Part model, mm, in its own coordinate system. A direction names the side the tool comes from. Round coordinates to 2 decimals unless told otherwise and drop trailing zeros. Loops run counter-clockwise (first coordinate to the right, second up) from the corner with the lowest first, then second, coordinate; pieces in that order, holes last.
from build123d import *

# Parameters (mm, degrees)
BOSS_EXTRUDE1_DEPTH = 6.35


with BuildPart() as part:
    # Sketch1 → Boss-Extrude1 (new body)
    with BuildSketch(Plane(origin=(0, 0, 0), x_dir=(1, 0, 0), z_dir=(0, 1, 0))):
        with BuildLine():
            Line((-79.362966154, -13.293541536), (-79.362966154, -21.341955347))
            Line((-79.362966154, -21.341955347), (-76.187966154, -21.341955347))
            Line((-76.187966154, -21.341955347), (-76.187966154, -19.589355347))
            Line((-76.187966154, -19.589355347), (-73.647966154, -19.589355347))
            Line((-73.647966154, -19.589355347), (-73.647966154, -21.341955347))
            Line((-73.647966154, -21.341955347), (-72.377966154, -21.341955347))
            Line((-72.377966154, -21.341955347), (-72.377966154, -24.389814703))
            Line((-72.377966154, -24.389814703), (-73.647966154, -24.389814703))
            Line((-73.647966154, -24.389814703), (-73.647966154, -26.142414703))
            Line((-73.647966154, -26.142414703), (-76.187966154, -26.142414703))
            Line((-76.187966154, -26.142414703), (-76.187966154, -24.389814703))
            Line((-76.187966154, -24.389814703), (-79.362966154, -24.389814703))
            Line((-79.362966154, -24.389814703), (-79.362966154, -32.343541536))
            Line((-79.362966154, -32.343541536), (-85.712966154, -32.343541536))
            Line((-85.712966154, -32.343541536), (-85.712966154, -38.693541536))
            Line((-85.712966154, -38.693541536), (-79.362966154, -38.693541536))
            Line((-79.362966154, -38.693541536), (-47.528264268, -38.693541536))
            Line((-47.528264268, -38.693541536), (-47.528264268, -35.518541536))
            Line((-47.528264268, -35.518541536), (-49.280864268, -35.518541536))
            Line((-49.280864268, -35.518541536), (-49.280864268, -32.978541536))
            Line((-49.280864268, -32.978541536), (-47.528264268, -32.978541536))
            Line((-47.528264268, -32.978541536), (-47.528264268, -31.708541536))
            Line((-47.528264268, -31.708541536), (-44.480404912, -31.708541536))
            Line((-44.480404912, -31.708541536), (-44.480404912, -32.978541536))
            Line((-44.480404912, -32.978541536), (-42.727804912, -32.978541536))
            Line((-42.727804912, -32.978541536), (-42.727804912, -35.518541536))
            Line((-42.727804912, -35.518541536), (-44.480404912, -35.518541536))
            Line((-44.480404912, -35.518541536), (-44.480404912, -38.693541536))
            Line((-44.480404912, -38.693541536), (20.734235732, -38.693541536))
            Line((20.734235732, -38.693541536), (20.734235732, -35.518541536))
            Line((20.734235732, -35.518541536), (18.981635732, -35.518541536))
            Line((18.981635732, -35.518541536), (18.981635732, -32.978541536))
            Line((18.981635732, -32.978541536), (20.734235732, -32.978541536))
            Line((20.734235732, -32.978541536), (20.734235732, -31.708541536))
            Line((20.734235732, -31.708541536), (23.782095088, -31.708541536))
            Line((23.782095088, -31.708541536), (23.782095088, -32.978541536))
            Line((23.782095088, -32.978541536), (25.534695088, -32.978541536))
            Line((25.534695088, -32.978541536), (25.534695088, -35.518541536))
            Line((25.534695088, -35.518541536), (23.782095088, -35.518541536))
            Line((23.782095088, -35.518541536), (23.782095088, -38.693541536))
            Line((23.782095088, -38.693541536), (79.387033846, -38.693541536))
            ThreePointArc((79.387033846, -38.693541536), (1.583968625, -14.958867645), (-79.362966154, -6.943541536))
            Line((-79.362966154, -6.943541536), (-85.712966154, -6.943541536))
            Line((-85.712966154, -6.943541536), (-85.712966154, -13.293541536))
            Line((-85.712966154, -13.293541536), (-79.362966154, -13.293541536))
        make_face()
    extrude(amount=BOSS_EXTRUDE1_DEPTH)


solid = part.part
1) Slice it at B-B, the plane z = 10. Give the cut face in (x, y), then the cut area to 3 significant figures.
Values:
outline: (-85.71, 0) - (-29.23, 0) - (-29.23, 6.35) - (-85.71, 6.35) - close
area: 359 mm2
2) Drop flat-ended pins along their axis: pin 1 Ø1.9 at (y, z) = (2.5, 20.5) entering from -X; pin 2 Ø1.5 at (y, z) = (2.5, 23) entering from -X; pin 3 Ø0.5 at (x, y) = (24.5, 4.5) entering from -Z. Give the stop position or say it passes through.
Values:
pin 1: stops at x = -79.36
pin 2: stops at x = -72.38
pin 3: stops at z = 20.16
3) Mould opens along X. For faces 5 (the face through (-79.363, 3, 17)), 6 (the face through (-47.528, 3, 37)), 7 (the face through (-23, 0, 26)) say: released by +X, released by -X, zero draft, split by the parting line, or undercut.
Values:
face 5: released by -X
face 6: undercut
face 7: zero draft
4) Slice it at A-A, the plane x = 11.5. Give the cut face in (y, z), then the cut area to 3 significant figures.
Values:
outline: (0, 17.07) - (6.35, 17.07) - (6.35, 38.69) - (0, 38.69) - close
area: 137 mm2
5) Tool access for faces 1 (the face through (-75, 3, 26.142)), 2 (the face through (-46, 3, 31.709)), 3 (the face through (-78, 3, 21.342)), 4 (the face through (-85.713, 3, 35)): list every direction of +Z, -Z, +X, -X, +Y, -Y with a clear straight run to the whole face (end or side of a thin tool).
Values:
face 1: +Y, -Y
face 2: +Z, +Y, -Y
face 3: -X, +Y, -Y
face 4: +Z, -Z, -X, +Y, -Y
6) Wall check: line 1 along Z through (x, y) = (-44, 2.75); line 2 along Z through (x, y) = (56, 1.75); line 3 along Z through (x, y) = (72.5, 4.5). Give the ranges that are in metal, low to high.
Values:
line 1: z = 8.46 to 32.98, 35.52 to 38.69
line 2: z = 29.77 to 38.69
line 3: z = 35.9 to 38.69
